Could you check a few things on this model? Use its own coordinates, in mm. A direction names the side the tool comes from. Give positions to 0.01 mm unless a question says otherwise; leave off trailing zeros. Loops run counter-clockwise (first coordinate to the right, second up) from the corner with the lowest first, then second, coordinate; pieces in that order, holes last.
1. For P1, Ø1.5, axis at x = 2, y = 1, coming from the -Z side; P2, Ø3, axis at x = 5.53, z = -19.58, coming from the -Y side; P3, Ø0.5, axis at y = 1.5, z = -38.5, coming from the -X side; P4, Ø1.6, axis at x = -28, y = 1, coming from the -Z side, each with a flat end and sliding along its axis, tell me the tip position at first contact or that it passes through.
2. Imagine slicing it at B-B (y = 3.05). List the corners of the cut face in (x, z) for me, plus the area to 3 significant figures.
3. I need wall thicknesses on line 1 along Z through (x, y) = (-11, 3.4); line 2 along Z through (x, y) = (-22, 1.15); line 3 along Z through (x, y) = (-6, 0.85). Which ranges of each line are inside material? Lowest first, please.
4. Imagine slicing it at A-A (x = -6). List the corners of the cut face in (y, z) for me.
5. Imagine slicing it at C-C (z = -7). List the corners of the cut face in (x, y) for me.
6. For faces 1 (the flat face through (5, 1, -38)), 2 (the flat face through (-27, 1, -8)), 3 (the flat face through (13.922, 0.76, -30.522)), 4 (the flat face through (-10, 3, -36.5)), which set-ups out of +Z, -Z, +X, -X, +Y, -Y let a thin tool reach every point of the face, with its end or its side?
7. Imagine slicing it at D-D (z = -34). List the corners of the cut face in (x, y) for me.
8. Thinking about a two-plate mould opening in Z: for faces 5 (the flat face through (-9.8, 4, -38.5)), 6 (the flat face through (-10, 3, -38)), 7 (the flat face through (8.465, 0.74, -14.662)), which applies, +Z half, -Z half, draft (parallel to the pull), parting line (faces both ways), or undercut?
Autodesk Inventor part; units mm, degrees
ref_plane "YZ Plane" through (0, 0, 0) normal (1, 0, 0) x (0, 1, 0)
ref_plane "XZ Plane" through (0, 0, 0) normal (0, 1, 0) x (-1, 0, 0)
ref_plane "XY Plane" through (0, 0, 0) normal (0, 0, 1) x (1, 0, 0)
sketch "スケッチ1" plane through (0, 0, 0) normal (0, 1, 0) x (-1, 0, 0)
  line L0 (0, 0) -> (30, 0)
  line L1 (30, 0) -> (30, -135.2775)
  line L2 (30, -135.2775) -> (-78.1025, -135.2775)
  line L3 (-78.1025, -135.2775) -> (0, 0)
  dimension "d0" = 30
  dimension "d1" = 60
extrude "押し出し1" add sketch "スケッチ1" along normal blind 1.5
sketch "スケッチ2" plane through (0, 1.5, 0) normal (0, 1, 0) x (1, 0, 0)
  line L0 (-25, 8) -> (-25, 1.5)
  line L1 (-21.9199, 13.3349) -> (-25, 8)
  line L2 (-30, 18) -> (-21.9199, 13.3349)
  line L3 (-24.2265, 28) -> (-30, 18)
  line L4 (0, 28) -> (-24.2265, 28)
  line L5 (0, 36.5) -> (0, 28)
  line L6 (5, 36.5) -> (0, 36.5)
  line L7 (5, 38) -> (5, 36.5)
  line L8 (10.9697, 38) -> (5, 38)
  line L9 (13.5677, 36.5) -> (10.9697, 38)
  line L10 (11.0677, 32.1699) -> (13.5677, 36.5)
  line L11 (16.6969, 28.9199) -> (11.0677, 32.1699)
  line L12 (7.3612, 12.75) -> (16.6969, 28.9199)
  line L13 (0, 17) -> (7.3612, 12.75)
  line L14 (-12, 17) -> (0, 17)
  line L15 (-12, 8) -> (-12, 17)
  line L16 (-5, 8) -> (-12, 8)
  line L17 (-5, 1.5) -> (-5, 8)
  line L18 (-25, 1.5) -> (-5, 1.5)
  line L19 (78.1025, 135.2775) -> (-30, 135.2775)
  line L20 (-30, 135.2775) -> (-30, 0)
  line L21 (-30, 0) -> (0, 0)
  line L22 (0, 0) -> (78.1025, 135.2775)
  line L23 (-24.2265, 28) -> (-18.453, 38)
  line L24 (-18.453, 38) -> (5, 38)
  line L25 (13.5677, 36.5) -> (19.1969, 33.25)
extrude "押し出し2" cut sketch "スケッチ2" against normal through all contours L20 L19 L22 L25 L9 L8 L24 L23 L3
sketch "スケッチ3" plane through (0, 1.5, 0) normal (0, 1, 0) x (1, 0, 0)
  line L0 (-30, 18) -> (-21.9199, 13.3349)
  line L1 (-21.9199, 13.3349) -> (-25, 8)
  line L2 (-25, 8) -> (-30, 8)
  line L3 (-30, 18) -> (-30, 0)
  line L4 (11.0677, 32.1699) -> (13.5677, 36.5)
  line L5 (16.6969, 28.9199) -> (11.0677, 32.1699)
  line L6 (19.1969, 33.25) -> (10.9697, 38)
  line L7 (0, 0) -> (19.1969, 33.25)
extrude "押し出し3" cut sketch "スケッチ3" against normal through all
sketch "スケッチ4" plane through (0, 0, 0) normal (0, -1, 0) x (1, 0, 0)
  line L0 (-18.453, -39) -> (3.9697, -39)
  line L1 (-18.453, -38) -> (-18.453, -39)
  line L2 (-18.453, -39) -> (3.9697, -39)
  line L3 (3.9697, -38) -> (-18.453, -38)
  line L4 (-1, -38) -> (-1, -36.5)
  line L5 (-1, -39) -> (-1, -35.5)
  line L6 (3.9697, -39) -> (3.9697, -38)
  line L7 (3.9697, -39) -> (3.9697, -38)
  line L8 (3.9697, -38) -> (-18.453, -38)
  line L9 (-18.453, -38) -> (-18.453, -39)
  line L10 (-18.453, -39) -> (3.9697, -39)
  line L11 (-1.0303, -36.5) -> (-1.0303, -35.5)
  line L12 (-1.0303, -35.5) -> (-18.453, -35.5)
  line L13 (-18.453, -35.5) -> (-18.453, -36.5)
  line L14 (-18.453, -36.5) -> (-1.0303, -36.5)
  point P0 (0, 0)
extrude "押し出し4" add sketch "スケッチ4" against normal blind 4 contours L1 L3 L5 L0 | L14 L13 L12 L11
sketch "スケッチ5" plane through (0, 0, 0) normal (0, -1, 0) x (1, 0, 0)
  circle A0 centre (-6, -23) radius 1.35
  circle A1 centre (5.5311, -19.5801) radius 1.35
  circle A2 centre (-16, -8) radius 1.35
  circle A3 centre (-22.5359, -22.9282) radius 1.35
  circle A4 centre (-22.5359, -22.9282) radius 1.6
  circle A5 centre (-16, -8) radius 1.6
  circle A6 centre (-6, -23) radius 1.6
  circle A7 centre (5.5311, -19.5801) radius 1.6
  point P0 (0, 0)
  dimension "d13" = 3.2
extrude "押し出し5" cut sketch "スケッチ5" against normal through all contours A0 | A1 | A2 | A3 | A4 | A5 | A6 | A7
equation "\"BendRadius\" = Thickness"
equation "\"BendReliefWidth\" = Thickness"
equation "\"BendReliefDepth\" = 0.5 * Thickness"
equation "\"CornerReliefSize\" = 4 * Thickness"
equation "\"MinimumRemnant\" = 2 * Thickness"
equation "\"TransitionRadius\" = BendRadius"
equation "\"JacobiRadiusSize\" = BendRadius"
equation "\"GapSize\" = Thickness"
equation "\"d6\" = Thickness"
properties part number "rail_cover_under"
Derived:
1. P1: stops at z = -38
1. P2: passes through
1. P3: stops at x = -18.45
1. P4: stops at z = -22.85
2. outline: (-18.45, -39) - (-1, -39) - (-1, -38) - (-18.45, -38) - close; (-18.45, -36.5) - (-1.03, -36.5) - (-1.03, -35.5) - (-18.45, -35.5) - close
2. area: 34.9 mm2
3. line 1: z = -39 to -38, -36.5 to -35.5
3. line 2: z = -31.86 to -24.44, -21.42 to -13.38, -13.2 to 0
3. line 3: z = -39 to -24.6, -21.4 to 0
4. outline: (0, -39) - (4, -39) - (4, -38) - (1.5, -38) - (1.5, -36.5) - (4, -36.5) - (4, -35.5) - (1.5, -35.5) - (1.5, -24.6) - (0, -24.6) - close; (0, -21.4) - (1.5, -21.4) - (1.5, 0) - (0, 0) - close
5. outline: (-30, 0) - (-17.25, 0) - (-17.25, 1.5) - (-30, 1.5) - close; (-14.75, 0) - (4.04, 0) - (4.04, 1.5) - (-14.75, 1.5) - close
6. face 1: -Z, +X, +Y, -Y
6. face 2: -X, +Y, -Y
6. face 3: +X, +Y, -Y
6. face 4: +X, -X, +Y
7. outline: (-20.76, 0) - (12.12, 0) - (12.12, 1.5) - (-20.76, 1.5) - close
8. face 5: draft
8. face 6: undercut
8. face 7: +Z half
